```python
from build123d import *

# Parameters (mm, degrees)
CROQUIS1_W              = 56
CROQUIS1_H              = 5
SALIENTE_EXTRUIR1_DEPTH = 12
CROQUIS2_R              = 4
SALIENTE_EXTRUIR2_DEPTH = 12
CROQUIS3_W              = 61.198456306
CROQUIS3_H              = 5.5
SALIENTE_EXTRUIR3_DEPTH = 12
CROQUIS4_R              = 2
CORTAR_EXTRUIR1_DEPTH   = 12
CROQUIS5_R              = 5
SALIENTE_EXTRUIR4_DEPTH = 12
CROQUIS6_W              = 56.358571572
CROQUIS6_H              = 7
SALIENTE_EXTRUIR5_DEPTH = 12
CROQUIS7_R              = 2
CORTAR_EXTRUIR2_DEPTH   = 12


with BuildPart() as part:
    # Croquis1 → Saliente-Extruir1 (new body)
    with BuildSketch(Plane(origin=(0, 0, 0), x_dir=(1, 0, 0), z_dir=(0, 1, 0))):
        Rectangle(CROQUIS1_W, CROQUIS1_H)
    extrude(amount=SALIENTE_EXTRUIR1_DEPTH)

    # Croquis2 → Saliente-Extruir2 (add)
    with BuildSketch(Plane(origin=(0, 12, 0), x_dir=(1, 0, 0), z_dir=(0, 1, 0))):
        with Locations((31.75, 0)):
            Circle(CROQUIS2_R)
        with Locations((-31.75, 0)):
            Circle(CROQUIS2_R)
    extrude(amount=-SALIENTE_EXTRUIR2_DEPTH)

    # Croquis3 → Saliente-Extruir3 (add)
    with BuildSketch(Plane(origin=(0, 12, 0), x_dir=(1, 0, 0), z_dir=(0, 1, 0))):
        Rectangle(CROQUIS3_W, CROQUIS3_H)
    extrude(amount=-SALIENTE_EXTRUIR3_DEPTH)

    # Croquis4 → Cortar-Extruir1 (cut)
    with BuildSketch(Plane(origin=(0, 12, 0), x_dir=(1, 0, 0), z_dir=(0, 1, 0))):
        with Locations((-31.75, 0)):
            Circle(CROQUIS4_R)
        with Locations((31.75, 0)):
            Circle(CROQUIS4_R)
    extrude(amount=-CORTAR_EXTRUIR1_DEPTH, mode=Mode.SUBTRACT)

    # Croquis5 → Saliente-Extruir4 (add)
    with BuildSketch(Plane(origin=(0, 12, 0), x_dir=(1, 0, 0), z_dir=(0, 1, 0))):
        with Locations((-31.75, 0)):
            Circle(CROQUIS5_R)
        with Locations((31.75, 0)):
            Circle(CROQUIS5_R)
    extrude(amount=-SALIENTE_EXTRUIR4_DEPTH)

    # Croquis6 → Saliente-Extruir5 (add)
    with BuildSketch(Plane(origin=(0, 12, 0), x_dir=(1, 0, 0), z_dir=(0, 1, 0))):
        Rectangle(CROQUIS6_W, CROQUIS6_H)
    extrude(amount=-SALIENTE_EXTRUIR5_DEPTH)

    # Croquis7 → Cortar-Extruir2 (cut)
    with BuildSketch(Plane(origin=(0, 12, 0), x_dir=(1, 0, 0), z_dir=(0, 1, 0))):
        with Locations((31.75, 0)):
            Circle(CROQUIS7_R)
        with Locations((-31.75, 0)):
            Circle(CROQUIS7_R)
    extrude(amount=-CORTAR_EXTRUIR2_DEPTH, mode=Mode.SUBTRACT)


solid = part.part
```
For this review, take the finished solid that the model builds, in its own axes (mm). A direction names the side the tool comes from. Round coordinates to 2 decimals unless told otherwise and drop trailing zeros. Write each loop counter-clockwise with the first axis right and the second up, starting at its lowest first coordinate (ties: lowest second). Pieces come first, ordered by that corner, then holes. Notation, with made-up numbers: (40.25, -22) -> (90.25, -22) arc R31 cw to (90.25, 13) -> close; hole circle Ø3 at (-12.5, 80.25). An arc over 180 degrees is marked (long way). One line per question, with ' | ' between items. Start each with the question number.
1) Wall thickness on line 1 along X through (y, z) = (1.25, -0.25); line 2 along Z through (x, y) = (-31.75, 3.25); line 3 along X through (y, z) = (2.75, -1.5): over which ranges is each line inside the solid? List them lowest first.
2) Add section C-C (y = 10.25). Write out the cut boundary in (x, z), and give its area (3 significant figures).
3) Mouldability with a two-part tool opening along Z and no side actions: class faces 3 (the flat face through (0, 6, 3.5)), 4 (the cylindrical face through (33.597, 6.084, 0.766)), 5 (the cylindrical face through (-36.747, 6.084, -0.166)) as +Z half, -Z half, draft (parallel to the pull), parting line (faces both ways), or undercut.
4) Add section B-B (z = 0). Write out the cut boundary in (x, y).
5) For pin 1 Ø1 at (x, y) = (-29, 8.5) entering from -Z; pin 2 Ø6 at (x, y) = (9.5, 7) entering from -Z; pin 3 Ø4 at (x, y) = (24.5, 3.5) entering from +Z, all flat-tipped, find the tip position at first contact; note any pin that passes through.
6) Add section A-A (x = -31.75). Write out the cut boundary in (y, z).
7) Machinability: for faces 1 (the flat face through (-1, 12, 0)), 2 (the flat face through (0, 6, -3.5)), which of the approach directions +Z, -Z, +X, -X, +Y, -Y give a long, thin tool a straight path to every point of the face, cutting with its end or side? Answer none if there is none.
8) Add section D-D (x = 12.5). Write out the cut boundary in (y, z).
Reported:
1) line 1: x = -36.74 to -33.73, -29.77 to 29.77, 33.73 to 36.74 | line 2: z = -5 to -2, 2 to 5 | line 3: x = -36.52 to -33.07, -30.43 to 30.43, 33.07 to 36.52
2) outline: (-28.18, -3.5) -> (28.18, -3.5) arc R5 ccw (long way) to (28.18, 3.5) -> (-28.18, 3.5) arc R5 ccw (long way) to start; hole circle Ø4 at (-31.75, 0); hole circle Ø4 at (31.75, 0) | area: 513 mm²
3) face 3: +Z half | face 4: undercut | face 5: parting line
4) outline: (-36.75, 0) -> (-33.75, 0) -> (-33.75, 12) -> (-36.75, 12) -> close; (-29.75, 0) -> (29.75, 0) -> (29.75, 12) -> (-29.75, 12) -> close; (33.75, 0) -> (36.75, 0) -> (36.75, 12) -> (33.75, 12) -> close
5) pin 1: stops at z = -4.47 | pin 2: stops at z = -3.5 | pin 3: stops at z = 3.5
6) outline: (0, -5) -> (12, -5) -> (12, -2) -> (0, -2) -> close; (0, 2) -> (12, 2) -> (12, 5) -> (0, 5) -> close
7) face 1: +Z, -Z, +X, -X, +Y | face 2: -Z, +Y, -Y
8) outline: (0, -3.5) -> (12, -3.5) -> (12, 3.5) -> (0, 3.5) -> close
